Can you work these out from the model? Positions are in its coordinate system, mm. Face numbers are marked on the shaded views. A direction names the side the tool comes from. Round coordinates to 2 decimals unless told otherwise and drop trailing zeros. Loops run counter-clockwise (first coordinate to the right, second up) from the corner with the lowest first, then second, coordinate; pieces in that order, holes last.
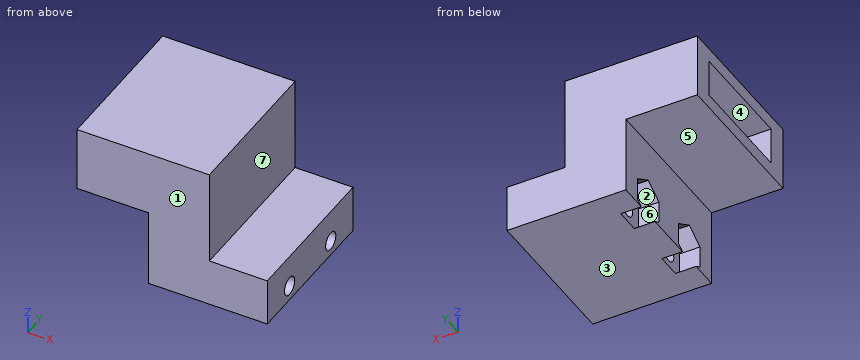
from build123d import *

# Parameters (mm, degrees)
BOSS_EXTRUDE1_DEPTH = 35.4
SKETCH2_W           = 8.63
SKETCH2_H           = 25.55
CUT_EXTRUDE1_DEPTH  = 30
SKETCH3_R           = 2.1
CUT_EXTRUDE2_DEPTH  = 64.958508207
CUT_EXTRUDE3_DEPTH  = 4.7625


with BuildPart() as part:
    # Sketch1 → Boss-Extrude1 (new body)
    with BuildSketch(Plane(origin=(0, 0, 0), x_dir=(1, 0, 0), z_dir=(0, 1, 0))):
        Polygon((1.0173917, 2.98), (-26.48, 2.98), (-26.48, -15), (-31.48, -15), (-43, -15), (-43, -30), (-12.38, -30), (-12.38, -8.02), (-11.48, -8.02), (1.0173917, -8.02), align=None)
    extrude(amount=BOSS_EXTRUDE1_DEPTH)

    # Sketch2 → Cut-Extrude1 (cut)
    with BuildSketch(Plane.ZY.offset(43)):
        with Locations((22.5, 17.7)):
            Rectangle(SKETCH2_W, SKETCH2_H)
    extrude(amount=-CUT_EXTRUDE1_DEPTH, mode=Mode.SUBTRACT)

    # Sketch3 → Cut-Extrude2 (cut, through all)
    with BuildSketch(Plane(origin=(1.0173917, 0, 0), x_dir=(0, 0, -1), z_dir=(1, 0, 0))):
        with Locations((-0.52, 9.2)):
            Circle(SKETCH3_R)
        with Locations((-0.52, 26.2)):
            Circle(SKETCH3_R)
    extrude(amount=-CUT_EXTRUDE2_DEPTH, mode=Mode.SUBTRACT)

    # Sketch4 → Cut-Extrude3 (cut)
    with BuildSketch(Plane.ZY.offset(26.48)):
        Polygon((-4.594313022, 9.2), (-2.037156511, 4.770875), (3.077156511, 4.770875), (5.634313022, 9.2), (3.077156511, 13.629125), (-2.037156511, 13.629125), align=None)
        Polygon((-4.594313022, 26.2), (-2.037156511, 21.770875), (3.077156511, 21.770875), (5.634313022, 26.2), (3.077156511, 30.629125), (-2.037156511, 30.629125), align=None)
    extrude(amount=-CUT_EXTRUDE3_DEPTH, mode=Mode.SUBTRACT)


solid = part.part
(1) If we section it at A-A, the plane z = 0.52: List the corners of the cut face in (x, y) for me.
Worked answers:
outline: (-26.48, 0) - (1.02, 0) - (1.02, 7.1) - (-21.72, 7.1) - (-21.72, 4.77) - (-26.48, 4.77) - close; (-26.48, 13.63) - (-21.72, 13.63) - (-21.72, 11.3) - (1.02, 11.3) - (1.02, 24.1) - (-21.72, 24.1) - (-21.72, 21.77) - (-26.48, 21.77) - close; (-26.48, 30.63) - (-21.72, 30.63) - (-21.72, 28.3) - (1.02, 28.3) - (1.02, 35.4) - (-26.48, 35.4) - close
(2) For the marked faces 5, 6 and 7, which set-ups out of +Z, -Z, +X, -X, +Y, -Y let a thin tool reach every point of the face, with its end or its side?
Worked answers:
face 5: -Z, -X, +Y, -Y
face 6: -X
face 7: +Z, +X, +Y, -Y
(3) If we section it at B-B, the plane x = -34.5: List the corners of the cut face in (y, z) for me (3 decimals), then the cut area to 3 significant figures.
Worked answers:
outline: (0, 15) - (35.4, 15) - (35.4, 30) - (0, 30) - close; hole (4.925, 18.185) - (30.475, 18.185) - (30.475, 26.815) - (4.925, 26.815) - close
area: 311 mm2
(4) If we section it at D-D, the plane x = -24: List the corners of the cut face in (y, z) for me (3 decimals).
Worked answers:
outline: (0, -2.98) - (6.404, -2.98) - (4.771, -2.037) - (4.771, 3.077) - (9.2, 5.634) - (13.629, 3.077) - (13.629, -2.037) - (11.996, -2.98) - (23.404, -2.98) - (21.771, -2.037) - (21.771, 3.077) - (26.2, 5.634) - (30.629, 3.077) - (30.629, -2.037) - (28.996, -2.98) - (35.4, -2.98) - (35.4, 30) - (0, 30) - close; hole (4.925, 18.185) - (30.475, 18.185) - (30.475, 26.815) - (4.925, 26.815) - close
(5) If we mould it in two halves opening along Z, with no side actions, what happens to the marked faces 1, 2, 3 and 4? For each: released by +Z, released by -Z, zero draft, split by the parting line, or undercut.
Worked answers:
face 1: zero draft
face 2: undercut
face 3: released by -Z
face 4: undercut
(6) Will these pins go through, and if not, where does the flat tip stop? P1, Ø7.5, axis at x = -35.5, y = 23, coming from the -Z side; P2, Ø4.5, axis at y = 26.5, z = -0.5, coming from the -X side; P3, Ø5.5, axis at y = 24.5, z = 6, coming from the -X side; P4, Ø4, axis at x = -24, z = -0.5, coming from the -Y side.
Worked answers:
P1: stops at z = 15
P2: stops at x = -21.72
P3: stops at x = -26.48
P4: stops at y = 0
(7) If we section it at C-C, the plane x = -2: List the corners of the cut face in (y, z) for me.
Worked answers:
outline: (0, -2.98) - (35.4, -2.98) - (35.4, 8.02) - (0, 8.02) - close; hole circle Ø4.2 at (9.2, 0.52); hole circle Ø4.2 at (26.2, 0.52)
(8) If I drill on line 1 (Y direction, x = -13, z = 0.52); line 2 (Y direction, x = -18, z = 21) (3 decimals); line 3 (Z direction, x = -16.5, y = 27) (3 decimals), over which ranges is the centre line in solid material (lowest first)?
Worked answers:
line 1: y = 0 to 7.1, 11.3 to 24.1, 28.3 to 35.4
line 2: y = 0 to 4.925, 30.475 to 35.4
line 3: z = -2.98 to -1.422, 2.462 to 18.185, 26.815 to 30
